Work out the finished part from the listing and answer in its coordinate system (mm). Face numbers are marked on the shaded views. A direction names the side the tool comes from. Coordinates: 2 decimals unless noted, no trailing zeros. Loops run counter-clockwise (first coordinate to the right, second up) from the corner with the lowest first, then second, coordinate; pieces in that order, holes last. Notation, with made-up numbers: (-27.5, -17.75) -> (13.5, -17.75) arc R37 ccw to (13.5, 19.25) -> close; hole circle Ø11 at (32.5, -11). An arc over 180 degrees is marked (long way). Use a Markdown table: item, result.
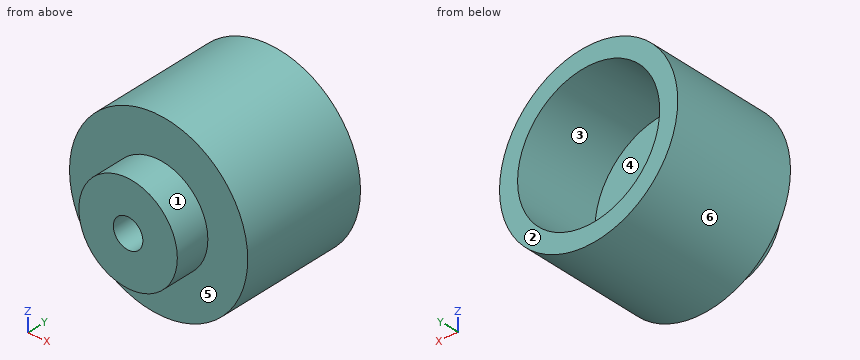
from build123d import *

# Parameters (mm, degrees)
ESQUISSE1_R             = 9.5
BOSS_EXTRU_2_DEPTH      = 13.3
ESQUISSE3_R             = 5.25
BOSS_EXTRU_3_DEPTH      = 3.6
ESQUISSE4_R             = 7.575
ENL_V_MAT_EXTRU_1_DEPTH = 9.13
ESQUISSE5_R             = 1.575
ENL_V_MAT_EXTRU_2_DEPTH = 9.13


with BuildPart() as part:
    # Esquisse1 → Boss.-Extru.2 (new body)
    with BuildSketch(Plane(origin=(0, 0, 0), x_dir=(1, 0, 0), z_dir=(0, 1, 0))):
        Circle(ESQUISSE1_R)
    extrude(amount=BOSS_EXTRU_2_DEPTH)

    # Esquisse3 → Boss.-Extru.3 (add)
    with BuildSketch(Plane.XZ):
        Circle(ESQUISSE3_R)
    extrude(amount=BOSS_EXTRU_3_DEPTH)

    # Esquisse4 → Enlèv. mat.-Extru.1 (cut)
    with BuildSketch(Plane(origin=(0, 13.3, 0), x_dir=(1, 0, 0), z_dir=(0, 1, 0))):
        Circle(ESQUISSE4_R)
    extrude(amount=-ENL_V_MAT_EXTRU_1_DEPTH, mode=Mode.SUBTRACT)

    # Esquisse5 → Enlèv. mat.-Extru.2 (cut)
    with BuildSketch(Plane.XZ.offset(3.6)):
        Circle(ESQUISSE5_R)
    extrude(amount=-ENL_V_MAT_EXTRU_2_DEPTH, mode=Mode.SUBTRACT)


solid = part.part
Q1. Section D-D on x = 4.75 is taken. Determine the outline of the cut face in (y, z), and give its area (3 significant figures).
Solved:
| item | result |
|---|---|
| outline | (-3.6, -2.24) -> (0, -2.24) -> (0, -8.23) -> (13.3, -8.23) -> (13.3, -5.9) -> (4.17, -5.9) -> (4.17, 5.9) -> (13.3, 5.9) -> (13.3, 8.23) -> (0, 8.23) -> (0, 2.24) -> (-3.6, 2.24) -> close |
| area | 127 mm² |
Q2. Section A-A on z = 0 is taken. Determine the outline of the cut face in (x, y) (3 decimals).
Solved:
| item | result |
|---|---|
| outline | (-9.5, 0) -> (-5.25, 0) -> (-5.25, -3.6) -> (-1.575, -3.6) -> (-1.575, 4.17) -> (-7.575, 4.17) -> (-7.575, 13.3) -> (-9.5, 13.3) -> close; (1.575, -3.6) -> (5.25, -3.6) -> (5.25, 0) -> (9.5, 0) -> (9.5, 13.3) -> (7.575, 13.3) -> (7.575, 4.17) -> (1.575, 4.17) -> close |
Q3. Determine the mould class of the marked faces 1, 2 and 3 for opening direction X: pulls with the +X half, pulls with the -X half, needs draft (parallel to the pull), parting line crosses it, or undercut.
Solved:
| item | result |
|---|---|
| face 1 | parting line crosses it |
| face 2 | needs draft |
| face 3 | undercut |
Q4. For the marked faces 4, 5 and 6, determine the directions among +Z, -Z, +X, -X, +Y, -Y from which every point of the face is accessible in a straight line to the end or side of a thin tool.
Solved:
| item | result |
|---|---|
| face 4 | +Y |
| face 5 | -Y |
| face 6 | +Y, -Y |
Q5. Given pin 1 Ø3 at (x, y) = (6, -2) entering from -Z; pin 2 Ø5 at (y, z) = (10.5, 6.5) entering from +X; pin 3 Ø1 at (y, z) = (2, -3.5) entering from +X, each flat-ended and moving along its own axis, determine where each tip first touches the part or whether it passes through.
Solved:
| item | result |
|---|---|
| pin 1 | z = -2.7 |
| pin 2 | x = 8.62 |
| pin 3 | x = 9.01 |
Q6. Section C-C on y = 6.75 is taken. Determine the outline of the cut face in (x, z) (3 decimals).
Solved:
| item | result |
|---|---|
| outline | circle Ø19 at (0, 0); hole circle Ø15.15 at (0, 0) |
Q7. Consider line 1 (Z direction, x = 0, y = 6) (3 decimals); line 2 (Y direction, x = 3, z = 5.5). Determine where each line is inside the solid, lowest interval first. Write a range as [from, to].
Solved:
| item | result |
|---|---|
| line 1 | [-9.5, -7.575], [7.575, 9.5] |
| line 2 | [0, 4.17] |
Q8. Section B-B on x = 0 is taken. Determine the outline of the cut face in (y, z) (3 decimals), and give its area (3 significant figures).
Solved:
| item | result |
|---|---|
| outline | (-3.6, -5.25) -> (0, -5.25) -> (0, -9.5) -> (13.3, -9.5) -> (13.3, -7.575) -> (4.17, -7.575) -> (4.17, -1.575) -> (-3.6, -1.575) -> close; (-3.6, 1.575) -> (4.17, 1.575) -> (4.17, 7.575) -> (13.3, 7.575) -> (13.3, 9.5) -> (0, 9.5) -> (0, 5.25) -> (-3.6, 5.25) -> close |
| area | 128 mm² |
